Verification items for the finished model (mm, model axes). A direction names the side the tool comes from. Round coordinates to 2 decimals unless told otherwise and drop trailing zeros. Loops run counter-clockwise (first coordinate to the right, second up) from the corner with the lowest first, then second, coordinate; pieces in that order, holes last.
from build123d import *

# Parameters (mm, degrees)
CROQUIS1_R              = 1.5
SALIENTE_EXTRUIR1_DEPTH = 2.5
SALIENTE_EXTRUIR2_START = -8.15
CROQUIS1_4_R            = 2.5
SALIENTE_EXTRUIR2_DEPTH = 7.87
SALIENTE_EXTRUIR3_DEPTH = 16.02
REDONDEO1_R             = 5
CROQUIS3_W              = 21.36
CROQUIS3_H              = 7.5
CROQUIS3_R              = 1.5
SALIENTE_EXTRUIR4_DEPTH = 2.5


with BuildPart() as part:
    # Croquis1 → Saliente-Extruir1 (new body)
    # profile 1 of 2: a face of its own
    with BuildSketch(Plane(origin=(0, 0, 0), x_dir=(1, 0, 0), z_dir=(0, 1, 0))):
        Polygon((3.6, 27.36), (-3.6, 27.36), (-3.6, 19.208695338), (3.6, 12.25573616), align=None)
        with Locations(Location((-0.4, 21.36, 0), (0, 0, 270))):
            Circle(CROQUIS1_R, mode=Mode.SUBTRACT)
    # profile 2 of 2: a face of its own
    with BuildSketch(Plane(origin=(0, 0, 0), x_dir=(1, 0, 0), z_dir=(0, 1, 0))):
        Polygon((3.6, 12.25573616), (-3.6, 19.208695338), (-3.6, 12.952959179), (3.6, 6), align=None)
    extrude(amount=-SALIENTE_EXTRUIR1_DEPTH)



with BuildPart() as body_2:
    # Croquis1<4> → Saliente-Extruir2 (new body)
    with BuildSketch(Plane(origin=(0, 0, 0), x_dir=(1, 0, 0), z_dir=(0, 1, 0)).offset(SALIENTE_EXTRUIR2_START)):
        with BuildLine():
            Line((3.6, 6), (-3.6, 12.952959179))
            Line((-3.6, 12.952959179), (-3.6, 0))
            ThreePointArc((-3.6, 0), (0, -3.6), (3.6, 0))
            Line((3.6, 0), (3.6, 6))
        make_face()
        with Locations(Location((0, 0, 0), (0, 0, 270))):
            Circle(CROQUIS1_4_R, mode=Mode.SUBTRACT)
    extrude(amount=-SALIENTE_EXTRUIR2_DEPTH)


with BuildPart() as part_1:
    add(part.part)

    add(body_2.part)  # Saliente-Extruir3 merges body 2
    # Croquis1<5> → Saliente-Extruir3 (add)
    with BuildSketch(Plane(origin=(0, 0, 0), x_dir=(1, 0, 0), z_dir=(0, 1, 0))):
        Polygon((3.6, 12.25573616), (-3.6, 19.208695338), (-3.6, 12.952959179), (3.6, 6), align=None)
    extrude(amount=-SALIENTE_EXTRUIR3_DEPTH)

    # Redondeo1
    redondeo1_edges = [part_1.edges().sort_by_distance(p)[0] for p in [
        (0, -16.02, -15.732215749),
    ]]
    fillet(redondeo1_edges, radius=REDONDEO1_R)

    # Croquis3 → Saliente-Extruir4 (add)
    # profile 1 of 2: a face of its own
    with BuildSketch(Plane(origin=(3.6, 0, 0), x_dir=(0, 0, -1), z_dir=(1, 0, 0))):
        with BuildLine():
            Line((6, 0), (6, -8.15))
            Line((6, -8.15), (6, -15.994937186))
            add(Edge.make_bspline(
                [(6, -15.994937186), (12.25573616, -15.542670169), (12.25573616, -11.02)],
                knots=[4.821475205, 4.821475205, 4.821475205, 6.283185307, 6.283185307, 6.283185307], degree=2, weights=[0.962144349, 0.727447175, 1]))
            Line((12.25573616, -11.02), (12.25573616, -2.5))
            Line((12.25573616, -2.5), (27.36, -2.5))
            Line((27.36, -2.5), (27.36, 0))
            Line((27.36, 0), (6, 0))
        make_face()
    # profile 2 of 2: a face of its own
    with BuildSketch(Plane(origin=(3.6, 0, 0), x_dir=(0, 0, -1), z_dir=(1, 0, 0))):
        with Locations((16.68, 3.75)):
            Rectangle(CROQUIS3_W, CROQUIS3_H)
        with Locations((11.36, 3.5)):
            Circle(CROQUIS3_R, mode=Mode.SUBTRACT)
    extrude(amount=SALIENTE_EXTRUIR4_DEPTH)


solid = part_1.part
1. Gauge pin test, flat ends, axial feed: P1, Ø5, axis at y = -11, z = -3, coming from the +X side; P2, Ø2, axis at x = 1.5, z = -6, coming from the +Y side; P3, Ø2.5, axis at x = -0.4, z = -21.36, coming from the +Y side; P4, Ø1.2, axis at x = 5, y = -6, coming from the -Z side. Record the tip position at first contact, or that the pin passes through.
2. Scan lines: L1, parallel to X at y = -11, z = 0; L2, parallel to Y at x = 4.25, z = -20; L3, parallel to X at y = -1.9, z = -21.36. Record each from-to range of solid material in increasing order.
3. Section check A-A (z = -21.36). Enter the section's corners in (x, y), then the cut area to 3 significant figures.
4. Section check B-B (y = 4). Enter the section's corners in (x, z), then the cut area to 3 significant figures.
5. Section check C-C (x = 0.5). Give the number of separate pieces and of enclosed holes in the cut face, then the cut area to 3 significant figures.
6. Release check for a two-part mould opening along Y. For faces 1 (the face through (0, 0, -19)), 2 (the face through (4.832, 2.925, -12.746)), 3 (the face through (0.05, -1.23, -19.93)), 4 (the face through (0.62, -14.59, -13.05)) record: released by +Y, released by -Y, zero draft, split by the parting line, or undercut.
7. Tool access check on faces 5 (the face through (3.6, 4, -17)), 6 (the face through (0.05, -6.7, -15.684)), 7 (the face through (3.6, -12, -3)), 8 (the face through (-1, -8.15, -5)). Record the directions out of +Z, -Z, +X, -X, +Y, -Y that give a thin tool (end or side, any length) a straight path to the whole face; none if there is none.
Taken from the geometry:
1. P1: stops at x = 3.6
1. P2: stops at y = -8.15
1. P3: passes through
1. P4: stops at z = -12.26
2. L1: x = -3.6 to -2.5, 2.5 to 3.6
2. L2: y = -2.5 to 7.5
2. L3: x = -3.6 to -1.9, 1.1 to 6.1
3. outline: (-3.6, -2.5) - (-1.9, -2.5) - (-1.9, 0) - (-3.6, 0) - close; (1.1, -2.5) - (6.1, -2.5) - (6.1, 7.5) - (3.6, 7.5) - (3.6, 0) - (1.1, 0) - close
3. area: 35.5 mm2
4. outline: (3.6, -27.36) - (6.1, -27.36) - (6.1, -12.77) - (3.6, -12.77) - close; (3.6, -9.95) - (6.1, -9.95) - (6.1, -6) - (3.6, -6) - close
4. area: 46.3 mm2
5. separate pieces: 3
5. enclosed holes: 0
5. area: 177 mm2
6. face 1: released by +Y
6. face 2: undercut
6. face 3: zero draft
6. face 4: released by -Y
7. face 5: +Z, -Z, -X, +Y
7. face 6: -Z, +X, -Y
7. face 7: +Z, +X, +Y, -Y
7. face 8: +Z, -X, +Y
